Can you work these out from the model? Positions are in its coordinate system, mm. A direction names the side the tool comes from. Coordinates: 2 decimals unless noted, no trailing zeros. Order: outer loops, then holes, each group sorted by start corner. A loop starts at its lowest first (then second) coordinate and runs counter-clockwise, first axis right, second up. Notation, with made-up numbers: (-23.75, 88) -> (-3.75, 88) arc R12 ccw to (-3.75, 93) -> close; hole circle Ø8 at (82, -35.75). An arc over 180 degrees is marked (long way). Write item = value, one per line.
```python
from build123d import *

# Parameters (mm, degrees)
SKETCH1_W           = 493
SKETCH1_H           = 355
BOSS_EXTRUDE1_DEPTH = 275
SKETCH2_W           = 40
SKETCH2_H           = 200
BOSS_EXTRUDE2_DEPTH = 38
CHAMFER1_SIZE       = 30


with BuildPart() as part:
    # Sketch1 → Boss-Extrude1 (new body)
    with BuildSketch(Plane(origin=(0, 0, 0), x_dir=(1, 0, 0), z_dir=(0, 1, 0))):
        Rectangle(SKETCH1_W, SKETCH1_H)
    extrude(amount=BOSS_EXTRUDE1_DEPTH)

    # Sketch2 → Boss-Extrude2 (add)
    with BuildSketch(Plane.XY.offset(177.5)):
        with Locations((150.868479839, 137.5)):
            Rectangle(SKETCH2_W, SKETCH2_H)
    extrude(amount=BOSS_EXTRUDE2_DEPTH)

    # Chamfer1
    chamfer1_edges = [part.edges().sort_by_distance(p)[0] for p in [
        (150.868479839, 37.5, 215.5),
        (150.868479839, 237.5, 215.5),
    ]]
    chamfer(chamfer1_edges, length=CHAMFER1_SIZE)


solid = part.part
```
Item 1: For faces 1 (the flat face through (170.868, 136, 196)), 2 (the flat face through (130.868, 136, 196)), 3 (the flat face through (151, 53, 201)), which set-ups out of +Z, -Z, +X, -X, +Y, -Y let a thin tool reach every point of the face, with its end or its side?
A:
face_1 = +Z, +X, +Y, -Y
face_2 = +Z, -X, +Y, -Y
face_3 = +Z, +X, -X, -Y
Item 2: I want a section at D-D, the plane x = 24. Please give me the cut outline in (y, z), plus the area to 3 significant figures.
A:
outline = (0, -177.5) -> (275, -177.5) -> (275, 177.5) -> (0, 177.5) -> close
area = 97,600 mm2
Item 3: I want a section at B-B, the plane x = 163.5. Please give me the cut outline in (y, z).
A:
outline = (0, -177.5) -> (275, -177.5) -> (275, 177.5) -> (237.5, 177.5) -> (237.5, 185.5) -> (207.5, 215.5) -> (67.5, 215.5) -> (37.5, 185.5) -> (37.5, 177.5) -> (0, 177.5) -> close
Item 4: If I drill on probe 1 along Z at (x, y) = (192, 135); probe 2 along Y at (x, z) = (150, 195), over which ranges is the centre line in solid material (lowest first)?
A:
probe_1 = -177.5 to 177.5
probe_2 = 47 to 228
Item 5: I want a section at A-A, the plane y = 227. Please give me the cut outline in (x, z).
A:
outline = (-246.5, -177.5) -> (246.5, -177.5) -> (246.5, 177.5) -> (170.87, 177.5) -> (170.87, 196) -> (130.87, 196) -> (130.87, 177.5) -> (-246.5, 177.5) -> close
Item 6: I want a section at C-C, the plane y = 168. Please give me the cut outline in (x, z), plus the area to 3 significant figures.
A:
outline = (-246.5, -177.5) -> (246.5, -177.5) -> (246.5, 177.5) -> (170.87, 177.5) -> (170.87, 215.5) -> (130.87, 215.5) -> (130.87, 177.5) -> (-246.5, 177.5) -> close
area = 177,000 mm2
Item 7: I'm going to push flat-ended pins straight in: P1, Ø9, axis at x = 146.5, z = 180, coming from the +Y side; P2, Ø2.5, axis at x = 153, z = 180, coming from the -Y side; P3, Ø11.5, axis at y = 165, z = 189, coming from the +X side; P4, Ø6, axis at x = -145, y = 246, coming from the +Z side. Where does each tip first touch, or does it pass through?
A:
P1 = 275
P2 = 37.5
P3 = 170.87
P4 = 177.5
